Source: CAD feature listing. Evaluate the final solid. Frame: model axes, mm. Face numbers are marked on the shaded views. A direction names the side the tool comes from. Coordinates: 2 decimals unless noted, no trailing zeros. Loops run counter-clockwise (first coordinate to the right, second up) from the corner with the lowest first, then second, coordinate; pieces in that order, holes last. Notation, with made-up numbers: (59.5, 9.5) -> (113.5, 9.5) arc R3 cw to (113.5, 13.5) -> close; hole circle Ø8 at (16.5, 32). An arc over 180 degrees is marked (long way). Answer as a JSON object with one key per item and string values. Group by question number.
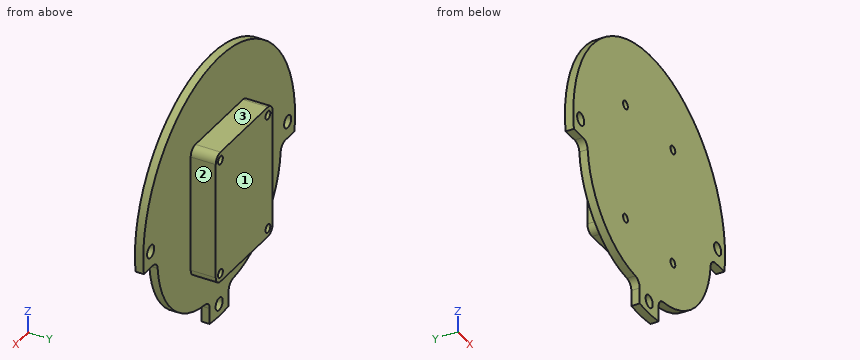
from build123d import *

# Parameters (mm, degrees)
SKETCH1_R           = 3.175
BOSS_EXTRUDE1_DEPTH = 25.4
SKETCH1_3_R         = 4.7625
BOSS_EXTRUDE2_DEPTH = 6.35


with BuildPart() as part:
    # Sketch1 → Boss-Extrude1 (new body)
    with BuildSketch(Plane(origin=(0, 0, 0), x_dir=(1, 0, 0), z_dir=(0, 1, 0))):
        with BuildLine():
            Line((-31.75, 50.8), (31.75, 50.8))
            ThreePointArc((31.75, 50.8), (36.240128061, 48.940128061), (38.1, 44.45))
            Line((38.1, 44.45), (38.1, -44.45))
            ThreePointArc((38.1, -44.45), (36.240128061, -48.940128061), (31.75, -50.8))
            Line((31.75, -50.8), (-31.75, -50.8))
            ThreePointArc((-31.75, -50.8), (-36.240128061, -48.940128061), (-38.1, -44.45))
            Line((-38.1, -44.45), (-38.1, 44.45))
            ThreePointArc((-38.1, 44.45), (-36.240128061, 48.940128061), (-31.75, 50.8))
        make_face()
        with Locations((31.75, -44.45)):
            Circle(SKETCH1_R, mode=Mode.SUBTRACT)
        with Locations((-31.75, -44.45)):
            Circle(SKETCH1_R, mode=Mode.SUBTRACT)
        with Locations((31.75, 44.45)):
            Circle(SKETCH1_R, mode=Mode.SUBTRACT)
        with Locations((-31.75, 44.45)):
            Circle(SKETCH1_R, mode=Mode.SUBTRACT)
    extrude(amount=BOSS_EXTRUDE1_DEPTH)

    # Sketch1_3 → Boss-Extrude2 (add)
    with BuildSketch(Plane(origin=(0, 0, 0), x_dir=(1, 0, 0), z_dir=(0, 1, 0))):
        with BuildLine():
            ThreePointArc((-82.307042742, 18.520833333), (-62.091408666, 62.091408666), (-18.520833333, 82.307042742))
            ThreePointArc((-18.520833333, 82.307042742), (-14.376526542, 84.335985396), (-12.7, 88.634955719))
            Line((-12.7, 88.634955719), (-12.7, 100.803124952))
            ThreePointArc((-12.7, 100.803124952), (0, 101.6), (12.7, 100.803124952))
            Line((12.7, 100.803124952), (12.7, 88.634955719))
            ThreePointArc((12.7, 88.634955719), (14.376526542, 84.335985396), (18.520833333, 82.307042742))
            ThreePointArc((18.520833333, 82.307042742), (62.091408666, 62.091408666), (82.307042742, 18.520833333))
            ThreePointArc((82.307042742, 18.520833333), (84.335985396, 14.376526542), (88.634955719, 12.7))
            Line((88.634955719, 12.7), (100.803124952, 12.7))
            ThreePointArc((100.803124952, 12.7), (0, -101.6), (-100.803124952, 12.7))
            Line((-100.803124952, 12.7), (-88.634955719, 12.7))
            ThreePointArc((-88.634955719, 12.7), (-84.335985396, 14.376526542), (-82.307042742, 18.520833333))
        make_face()
        with Locations((91.676562476, 0)):
            Circle(SKETCH1_3_R, mode=Mode.SUBTRACT)
        with Locations((-91.676562476, 0)):
            Circle(SKETCH1_3_R, mode=Mode.SUBTRACT)
        with Locations((0, 92.075)):
            Circle(SKETCH1_3_R, mode=Mode.SUBTRACT)
        with BuildLine():
            ThreePointArc((-31.75, 50.8), (-36.240128061, 48.940128061), (-38.1, 44.45))
            Line((-38.1, 44.45), (-38.1, -44.45))
            ThreePointArc((-38.1, -44.45), (-36.240128061, -48.940128061), (-31.75, -50.8))
            Line((-31.75, -50.8), (31.75, -50.8))
            ThreePointArc((31.75, -50.8), (36.240128061, -48.940128061), (38.1, -44.45))
            Line((38.1, -44.45), (38.1, 44.45))
            ThreePointArc((38.1, 44.45), (36.240128061, 48.940128061), (31.75, 50.8))
            Line((31.75, 50.8), (-31.75, 50.8))
        make_face(mode=Mode.SUBTRACT)
    extrude(amount=BOSS_EXTRUDE2_DEPTH)


solid = part.part
1. Section query D-D on z = -56. Return loops of the section in (x, y).
2. Section query B-B on z = 0. Return loops of the section in (x, y).
3. Section query A-A on y = 16.5. Return loops of the section in (x, z) (3 decimals), then the cut area to 3 significant figures.
4. Section query C-C on x = -49.5. Return loops of the section in (y, z), then the cut area to 3 significant figures.
5. Pin query (flat end, axial travel): pin 1 Ø3 at (y, z) = (4.5, -96.5) entering from +X; pin 2 Ø1 at (y, z) = (23, -39.5) entering from -X; pin 3 Ø3 at (x, y) = (94, 2.5) entering from -Z. Return the tip coordinate at first contact, or that it passes through.
6. Ray query, L1, parallel to Z at x = 31.75, y = 13 (3 decimals); L2, parallel to Z at x = -29.5, y = 9.25; L3, parallel to X at y = 21.5, z = 43. Return the intervals inside material, ascending.
7. Reachability of the marked faces 1, 2 and 3 from +Z, -Z, +X, -X, +Y, -Y: full face, straight path, thin tool, end or side. Return the list, or none.
Solved:
{
 "1": {"outline": "(-67.51, 0) -> (67.51, 0) -> (67.51, 6.35) -> (-67.51, 6.35) -> close"},
 "2": {"outline": "(-101.6, 0) -> (-96.44, 0) -> (-96.44, 6.35) -> (-101.6, 6.35) -> close; (-86.91, 0) -> (86.91, 0) -> (86.91, 6.35) -> (38.1, 6.35) -> (38.1, 25.4) -> (-38.1, 25.4) -> (-38.1, 6.35) -> (-86.91, 6.35) -> close; (96.44, 0) -> (101.6, 0) -> (101.6, 6.35) -> (96.44, 6.35) -> close"},
 "3": {"outline": "(-38.1, -44.45) arc R6.35 ccw to (-31.75, -50.8) -> (31.75, -50.8) arc R6.35 ccw to (38.1, -44.45) -> (38.1, 44.45) arc R6.35 ccw to (31.75, 50.8) -> (-31.75, 50.8) arc R6.35 ccw to (-38.1, 44.45) -> close; hole circle Ø6.35 at (-31.75, -44.45); hole circle Ø6.35 at (-31.75, 44.45); hole circle Ø6.35 at (31.75, -44.45); hole circle Ø6.35 at (31.75, 44.45)", "area": "7,580 mm^2"},
 "4": {"outline": "(0, -72.07) -> (6.35, -72.07) -> (6.35, 88.73) -> (0, 88.73) -> close", "area": "1,020 mm^2"},
 "5": {"pin 1": "x = 12.7", "pin 2": "x = -38.1", "pin 3": "z = -12.7"},
 "6": {"L1": "-50.8 to -47.625, -41.275 to 41.275, 47.625 to 50.8", "L2": "-50.8 to -46.69, -42.21 to 42.21, 46.69 to 50.8", "L3": "-38.1 to -34.57, -28.93 to 28.93, 34.57 to 38.1"},
 "7": {"face 1": "+Z, -Z, +X, -X, +Y", "face 2": "+Z, -Z, +X, +Y", "face 3": "+Z, +X, -X, +Y"}
}
